Part model, mm, in its own coordinate system. Face numbers are marked on the shaded views. A direction names the side the tool comes from. Round coordinates to 2 decimals unless told otherwise and drop trailing zeros. Loops run counter-clockwise (first coordinate to the right, second up) from the corner with the lowest first, then second, coordinate; pieces in that order, holes last.
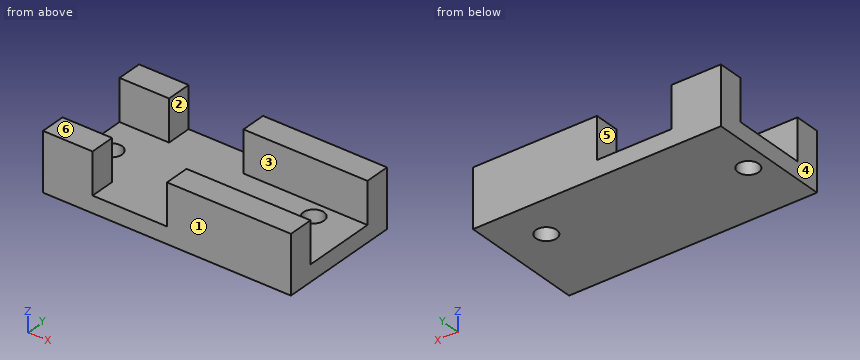
from build123d import *

# Parameters (mm, degrees)
SKETCH1_W           = 76.2
SKETCH1_H           = 38.1
BOSS_EXTRUDE1_DEPTH = 5.08
SKETCH2_W           = 38.1
SKETCH2_H           = 7.747
SKETCH2_W_2         = 15.24
BOSS_EXTRUDE2_DEPTH = 12.7
SKETCH3_R           = 3.175
CUT_EXTRUDE1_DEPTH  = 6.08
SKETCH4_R           = 3.175
CUT_EXTRUDE2_DEPTH  = 6.08


with BuildPart() as part:
    # Sketch1 → Boss-Extrude1 (new body)
    with BuildSketch(Plane.XY):
        Rectangle(SKETCH1_W, SKETCH1_H)
    extrude(amount=BOSS_EXTRUDE1_DEPTH)

    # Sketch2 → Boss-Extrude2 (add)
    with BuildSketch(Plane.XY.offset(5.08)):
        with Locations((19.05, 15.1765)):
            Rectangle(SKETCH2_W, SKETCH2_H)
        with Locations((19.05, -15.1765)):
            Rectangle(SKETCH2_W, SKETCH2_H)
        with Locations((-30.48, 15.1765)):
            Rectangle(SKETCH2_W_2, SKETCH2_H)
        with Locations((-30.48, -15.1765)):
            Rectangle(SKETCH2_W_2, SKETCH2_H)
    extrude(amount=BOSS_EXTRUDE2_DEPTH)

    # Sketch3 → Cut-Extrude1 (cut, through all)
    with BuildSketch(Plane.XY.offset(5.08)):
        with Locations((25.4, 6.35)):
            Circle(SKETCH3_R)
    extrude(amount=-CUT_EXTRUDE1_DEPTH, mode=Mode.SUBTRACT)

    # Sketch4 → Cut-Extrude2 (cut, through all)
    with BuildSketch(Plane.XY.offset(5.08)):
        with Locations((-31.75, 0)):
            Circle(SKETCH4_R)
    extrude(amount=-CUT_EXTRUDE2_DEPTH, mode=Mode.SUBTRACT)


solid = part.part
1) Slice it at B-B, the plane z = 8. Give the cut face in (x, y), then the cut area to 3 significant figures.
Values:
outline: (-38.1, -19.05) - (-22.86, -19.05) - (-22.86, -11.3) - (-38.1, -11.3) - close; (-38.1, 11.3) - (-22.86, 11.3) - (-22.86, 19.05) - (-38.1, 19.05) - close; (0, -19.05) - (38.1, -19.05) - (38.1, -11.3) - (0, -11.3) - close; (0, 11.3) - (38.1, 11.3) - (38.1, 19.05) - (0, 19.05) - close
area: 826 mm2
2) Slice it at C-C, the plane x = 25.4. Give the cut face in (y, z) (3 decimals).
Values:
outline: (-19.05, 0) - (3.175, 0) - (3.175, 5.08) - (-11.303, 5.08) - (-11.303, 17.78) - (-19.05, 17.78) - close; (9.525, 0) - (19.05, 0) - (19.05, 17.78) - (11.303, 17.78) - (11.303, 5.08) - (9.525, 5.08) - close
3) Drop flat-ended pins along their axis: pin 1 Ø5 at (x, z) = (-18, 14.5) entering from +Y; pin 2 Ø1 at (x, y) = (24, -8.5) entering from +Z. Give the stop position or say it passes through.
Values:
pin 1: passes through
pin 2: stops at z = 5.08
4) Tool access for the marked faces 1, 2 and 3: list every direction of +Z, -Z, +X, -X, +Y, -Y with a clear straight run to the whole face (end or side of a thin tool).
Values:
face 1: +Z, -Z, +X, -X, -Y
face 2: +Z, +Y, -Y
face 3: +Z, +X, -X
5) Mould opens along X. For the marked faces 4, 5 and 6 say: released by +X, released by -X, zero draft, split by the parting line, or undercut.
Values:
face 4: released by -X
face 5: undercut
face 6: zero draft
6) Slice it at D-D, the plane y = -15. Give the cut face in (x, z).
Values:
outline: (-38.1, 0) - (38.1, 0) - (38.1, 17.78) - (0, 17.78) - (0, 5.08) - (-22.86, 5.08) - (-22.86, 17.78) - (-38.1, 17.78) - close
7) Slice it at A-A, the plane y = 0. Give the cut face in (x, z) (3 decimals), then the cut area to 3 significant figures.
Values:
outline: (-38.1, 0) - (-34.925, 0) - (-34.925, 5.08) - (-38.1, 5.08) - close; (-28.575, 0) - (38.1, 0) - (38.1, 5.08) - (-28.575, 5.08) - close
area: 355 mm2
8) Wall check: line 1 along Y through (x, z) = (-31.75, 3.7) (3 decimals); line 2 along X through (y, z) = (12.5, 7.5); line 3 along Y through (x, z) = (30, 15.5). Give the ranges that are in metal, low to high.
Values:
line 1: y = -19.05 to -3.175, 3.175 to 19.05
line 2: x = -38.1 to -22.86, 0 to 38.1
line 3: y = -19.05 to -11.3, 11.3 to 19.05
